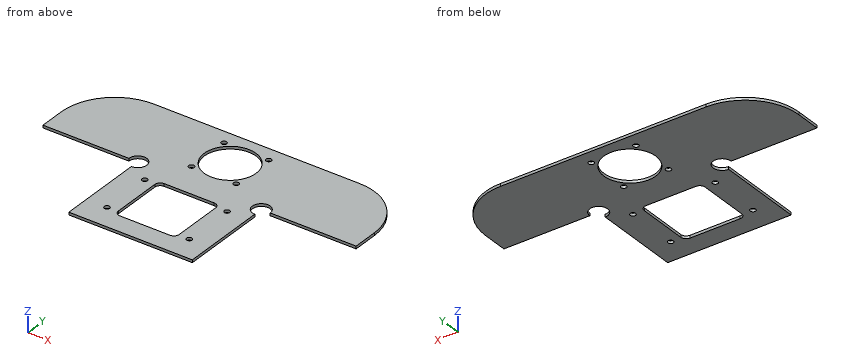
```python
from build123d import *

# Parameters (mm, degrees)
SKETCH_R   = 1.5
SKETCH_R_2 = 14.5
PAD_DEPTH  = 1.5


with BuildPart() as part:
    # Sketch → Pad (new body)
    with BuildSketch(Plane.XY):
        with BuildLine():
            Line((34.5, -45), (-34.5, -45))
            Line((-34.5, 3), (-34.5, -45))
            ThreePointArc((-34.5, 3), (-30.964466, 11.535534), (-39.5, 8))
            Line((-87.5, 8), (-39.5, 8))
            Line((-87.5, 22), (-87.5, 8))
            ThreePointArc((-57.5, 52), (-78.713203, 43.213203), (-87.5, 22))
            Line((57.5, 52), (-57.5, 52))
            ThreePointArc((87.5, 22), (78.713203, 43.213203), (57.5, 52))
            Line((87.5, 22), (87.5, 8))
            Line((87.5, 8), (39.5, 8))
            ThreePointArc((39.5, 8), (30.964466, 11.535534), (34.5, 3))
            Line((34.5, 3), (34.5, -45))
        make_face()
        with Locations((23, -2.5)):
            Circle(SKETCH_R, mode=Mode.SUBTRACT)
        with Locations((23, -31.5)):
            Circle(SKETCH_R, mode=Mode.SUBTRACT)
        with Locations((-23, -2.5)):
            Circle(SKETCH_R, mode=Mode.SUBTRACT)
        with Locations((-23, -31.5)):
            Circle(SKETCH_R, mode=Mode.SUBTRACT)
        with Locations((0, 31.5)):
            Circle(SKETCH_R_2, mode=Mode.SUBTRACT)
        with Locations((-12.5, 44)):
            Circle(SKETCH_R, mode=Mode.SUBTRACT)
        with Locations((12.5, 44)):
            Circle(SKETCH_R, mode=Mode.SUBTRACT)
        with Locations((12.5, 19)):
            Circle(SKETCH_R, mode=Mode.SUBTRACT)
        with Locations((-12.5, 19)):
            Circle(SKETCH_R, mode=Mode.SUBTRACT)
        with BuildLine():
            Line((-14, 0), (14, 0))
            ThreePointArc((17, -3), (16.12132, -0.87868), (14, 0))
            Line((17, -3), (17, -31))
            ThreePointArc((14, -34), (16.12132, -33.12132), (17, -31))
            Line((14, -34), (-14, -34))
            ThreePointArc((-17, -31), (-16.12132, -33.12132), (-14, -34))
            Line((-17, -31), (-17, -3))
            ThreePointArc((-14, 0), (-16.12132, -0.87868), (-17, -3))
        make_face(mode=Mode.SUBTRACT)
    extrude(amount=PAD_DEPTH)


solid = part.part
```
Part model, mm, in its own coordinate system. Coordinates: 2 decimals unless noted, no trailing zeros. Order: outer loops, then holes, each group sorted by start corner. A loop starts at its lowest first (then second) coordinate and runs counter-clockwise, first axis right, second up. Notation, with made-up numbers: (-24.75, 74) -> (2.25, 74) arc R17 cw to (2.25, 79) -> close; hole circle Ø8 at (59, 1.5). An arc over 180 degrees is marked (long way). Put each result on its own line as item: value. Start each with the question number.
(1) Band-saw the part on B-B (x = 0). Give the cut face in (y, z).
(2) Pin check, flat tip, straight feed: pin 1 Ø6 at (x, y) = (-34.5, 8) entering from +Z. Stop position of the tip, or through.
(3) Band-saw the part on C-C (y = -12). Give the cut face in (x, z), then the cut area to 3 significant figures.
(4) Band-saw the part on D-D (y = 39). Give the cut face in (x, z), then the cut area to 3 significant figures.
(5) Band-saw the part on A-A (z = 0.55). Count the separate pieces of the cut face and the enclosed holes in it, then the cut area to 3 significant figures.
(6) Probe line 1 along Y through (x, z) = (0, 0.3); line 2 along Y through (x, z) = (-12.5, 0.75); line 3 along X through (y, z) = (9.5, 0.2). List the from-to ranges inside material, lowest first. Write a range as [from, to].
Determined:
1. outline: (-45, 0) -> (-34, 0) -> (-34, 1.5) -> (-45, 1.5) -> close; (0, 0) -> (17, 0) -> (17, 1.5) -> (0, 1.5) -> close; (46, 0) -> (52, 0) -> (52, 1.5) -> (46, 1.5) -> close
2. pin 1: passes through
3. outline: (-34.5, 0) -> (-17, 0) -> (-17, 1.5) -> (-34.5, 1.5) -> close; (17, 0) -> (34.5, 0) -> (34.5, 1.5) -> (17, 1.5) -> close
3. area: 52.5 mm²
4. outline: (-82.22, 0) -> (-12.41, 0) -> (-12.41, 1.5) -> (-82.22, 1.5) -> close; (12.41, 0) -> (82.22, 0) -> (82.22, 1.5) -> (12.41, 1.5) -> close
4. area: 209 mm²
5. separate pieces: 1
5. enclosed holes: 10
5. area: 8,990 mm²
6. line 1: y = [-45, -34], [0, 17], [46, 52]
6. line 2: y = [-45, -34], [0, 17.5], [20.5, 24.15], [38.85, 42.5], [45.5, 52]
6. line 3: x = [-87.5, -39.27], [-29.73, 29.73], [39.27, 87.5]
